```python
from build123d import *

# Parameters (mm, degrees)
CROQUIS1_W              = 41
CROQUIS1_H              = 21
SALIENTE_EXTRUIR1_DEPTH = 4
CROQUIS2_W              = 12
CROQUIS2_H              = 21.062925544
CORTAR_EXTRUIR1_DEPTH   = 3
CROQUIS3_W              = 7
CROQUIS3_H              = 21
CORTAR_EXTRUIR2_DEPTH   = 3
CROQUIS4_OUTSIDE_W      = 52.248
CROQUIS4_OUTSIDE_H      = 32.248
CROQUIS4_OUTSIDE_W_2    = 22
CROQUIS4_OUTSIDE_H_2    = 13
CORTAR_EXTRUIR3_DEPTH   = 3
REDONDEO1_R             = 2
CROQUIS5_R              = 0.71529937
CORTAR_EXTRUIR5_DEPTH   = 3
MATRIZL2_COUNT          = 8
MATRIZL2_PITCH          = 2.4
CROQUIS6_R              = 1.5
CORTAR_EXTRUIR6_DEPTH   = 3
CROQUIS7_W              = 5.91959288
CROQUIS7_H              = 12.713547862
SALIENTE_EXTRUIR2_DEPTH = 0.5


with BuildPart() as part:
    # Croquis1 → Saliente-Extruir1 (new body)
    with BuildSketch(Plane(origin=(0, 0, 0), x_dir=(1, 0, 0), z_dir=(0, 1, 0))):
        Rectangle(CROQUIS1_W, CROQUIS1_H)
    extrude(amount=SALIENTE_EXTRUIR1_DEPTH)

    # Croquis2 → Cortar-Extruir1 (cut)
    with BuildSketch(Plane(origin=(0, 4, 0), x_dir=(1, 0, 0), z_dir=(0, 1, 0))):
        with Locations((-14.5, -0.031462772)):
            Rectangle(CROQUIS2_W, CROQUIS2_H)
    extrude(amount=-CORTAR_EXTRUIR1_DEPTH, mode=Mode.SUBTRACT)

    # Croquis3 → Cortar-Extruir2 (cut)
    with BuildSketch(Plane(origin=(0, 4, 0), x_dir=(1, 0, 0), z_dir=(0, 1, 0))):
        with Locations((17, 0)):
            Rectangle(CROQUIS3_W, CROQUIS3_H)
    extrude(amount=-CORTAR_EXTRUIR2_DEPTH, mode=Mode.SUBTRACT)

    # Croquis4 outside → Cortar-Extruir3 (cut)
    with BuildSketch(Plane(origin=(0, 4, 0), x_dir=(1, 0, 0), z_dir=(0, 1, 0))):
        Rectangle(CROQUIS4_OUTSIDE_W, CROQUIS4_OUTSIDE_H)
        with Locations((2.5, 0)):
            Rectangle(CROQUIS4_OUTSIDE_W_2, CROQUIS4_OUTSIDE_H_2, mode=Mode.SUBTRACT)
    extrude(amount=-CORTAR_EXTRUIR3_DEPTH, mode=Mode.SUBTRACT)

    # Redondeo1
    redondeo1_edges = [part.edges().sort_by_distance(p)[0] for p in [
        (-20.5, 0.5, 10.5),
        (-20.5, 0.5, -10.5),
        (20.5, 0.5, 10.5),
        (20.5, 0.5, -10.5),
    ]]
    fillet(redondeo1_edges, radius=REDONDEO1_R)

    # Croquis5 → Cortar-Extruir5 (cut)
    with BuildSketch(Plane(origin=(0, 1, 0), x_dir=(1, 0, 0), z_dir=(0, 1, 0))):
        with Locations((-18.975797273, -8.5)):
            Circle(CROQUIS5_R)
    cortar_extruir5 = extrude(amount=-CORTAR_EXTRUIR5_DEPTH, mode=Mode.SUBTRACT)

    # MatrizL2: Cortar-Extruir5 ×8
    with Locations(*[(0, 0, -i * MATRIZL2_PITCH) for i in range(1, MATRIZL2_COUNT)]):
        add(cortar_extruir5, mode=Mode.SUBTRACT)

    # Croquis6 → Cortar-Extruir6 (cut)
    with BuildSketch(Plane(origin=(0, 1, 0), x_dir=(1, 0, 0), z_dir=(0, 1, 0))):
        with Locations((-15.149962862, 8.506455595)):
            Circle(CROQUIS6_R)
        with Locations((18.5, 8.506455595)):
            Circle(CROQUIS6_R)
        with Locations((-15.149962862, -8.178172234)):
            Circle(CROQUIS6_R)
        with Locations((18.5, -8.178172234)):
            Circle(CROQUIS6_R)
    extrude(amount=-CORTAR_EXTRUIR6_DEPTH, mode=Mode.SUBTRACT)

    # Croquis7 → Saliente-Extruir2 (add)
    with BuildSketch(Plane(origin=(0, 1, 0), x_dir=(1, 0, 0), z_dir=(0, 1, 0))):
        with Locations((17.54020356, -0.02363113)):
            Rectangle(CROQUIS7_W, CROQUIS7_H)
    extrude(amount=SALIENTE_EXTRUIR2_DEPTH)


solid = part.part
```
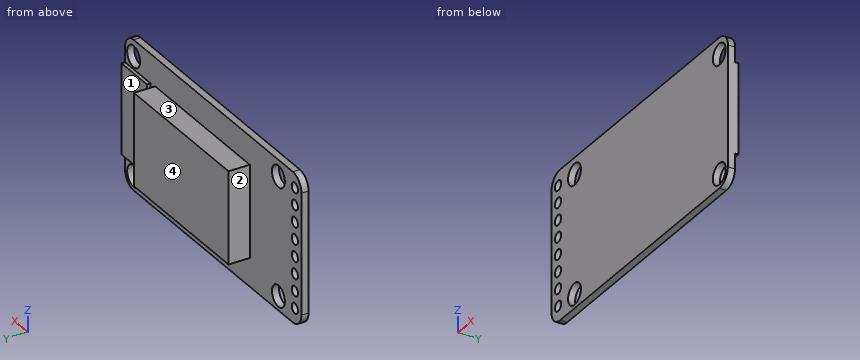
Source: CAD feature listing. Evaluate the final solid. Frame: model axes, mm. Face numbers are marked on the shaded views. A direction names the side the tool comes from. Coordinates: 2 decimals unless noted, no trailing zeros. Write each loop counter-clockwise with the first axis right and the second up, starting at its lowest first coordinate (ties: lowest second). Pieces come first, ordered by that corner, then holes. Notation, with made-up numbers: (-26.75, 72) - (-3.75, 72) arc R22 ccw to (-3.75, 108) - close; hole circle Ø4 at (63, -35). An arc over 180 degrees is marked (long way). Answer as a JSON object with one key per item and string values.
Q1. Material intervals for line 1 (X direction, y = 1.05, z = 4.25); line 2 (X direction, y = 0.4, z = -8.3); line 3 (Z direction, x = -7, y = 1.9), sorted ascending. Write a range as [from, to].
Ans:
{"line 1": "x = [-8.5, 13.5], [14.58, 20.5]", "line 2": "x = [-20.5, -19.69], [-18.26, -16.64], [-13.66, 17.01], [19.99, 20.5]", "line 3": "z = [-6.5, 6.5]"}
Q2. Section query B-B, the plane x = -4. Output: boundary loops of the cut face in (y, z).
Ans:
{"outline": "(0, -10.5) - (1, -10.5) - (1, -6.5) - (4, -6.5) - (4, 6.5) - (1, 6.5) - (1, 10.5) - (0, 10.5) - close"}
Q3. First-contact query: pin 1 Ø1.1 at (x, z) = (-18.98, 1.3) entering from +Y; pin 2 Ø5 at (x, z) = (18.5, -8.51) entering from +Y; pin 3 Ø0.9 at (x, y) = (4.5, 2) entering from -Z; pin 4 Ø1.9 at (x, z) = (-18.98, 6.1) entering from +Y. Flat tips, straight axial feed; report the tip coordinate or a pass-through.
Ans:
{"pin 1": "passes through", "pin 2": "stops at y = 1.5", "pin 3": "stops at z = -6.5", "pin 4": "stops at y = 1"}
Q4. Set-up query: the marked faces 1, 2, 3 and 4. Return all of +Z, -Z, +X, -X, +Y, -Y with unobstructed straight access to the full face (end or side cutting, diameter ignored); none if empty.
Ans:
{"face 1": "+Z, -Z, +X, +Y", "face 2": "+Z, -Z, -X, +Y", "face 3": "+Z, +X, -X, +Y", "face 4": "+Z, -Z, +X, -X, +Y"}
Q5. Section query A-A, the plane z = -5.9. Output: boundary loops of the cut face in (x, y).
Ans:
{"outline": "(-20.5, 0) - (-19.69, 0) - (-19.69, 1) - (-20.5, 1) - close; (-18.26, 0) - (20.5, 0) - (20.5, 1.5) - (14.58, 1.5) - (14.58, 1) - (13.5, 1) - (13.5, 4) - (-8.5, 4) - (-8.5, 1) - (-18.26, 1) - close"}
Q6. Section query C-C, the plane y = 0.6. State how many separate pieces and enclosed holes the cut face has, plus the area to 3 significant figures.
Ans:
{"separate pieces": "1", "enclosed holes": "12", "area": "816 mm2"}
Q7. Section query D-D, the plane y = 2.65. Output: boundary loops of the cut face in (x, z).
Ans:
{"outline": "(-8.5, -6.5) - (13.5, -6.5) - (13.5, 6.5) - (-8.5, 6.5) - close"}
